Could you check a few things on this model? Use its own coordinates, in mm. Face numbers are marked on the shaded views. A direction names the side the tool comes from. Give positions to 0.01 mm unless a question says otherwise; leave off trailing zeros. Order: outer loops, then holes, each group sorted by start corner. A loop starts at its lowest first (then second) coordinate and runs counter-clockwise, first axis right, second up. Notation, with made-up numbers: (82, -7.75) - (123, -7.75) arc R34 cw to (123, 31.25) - close; hole circle Ø11 at (-27, 17.5). An arc over 180 degrees is marked (long way). One line per question, with ' | ' between items. Start each with the question number.
1. Which directions (+Z, -Z, +X, -X, +Y, -Y) give clear straight access to the entire face, cutting with the end or side of a thin tool? Please do the marked faces 1 and 2.
2. Imagine slicing it at A-A (y = 39.5). Please give me the cut outline in (x, z), and give its area (3 significant figures).
3. Imagine slicing it at B-B (x = 6). Please give me the cut outline in (y, z).
4. For P1, Ø0.8, axis at x = 34, y = 10, coming from the -Z side; P2, Ø8.5, axis at x = 15, y = 15.5, coming from the -Z side; P3, Ø10, axis at y = 46.5, z = -2.5, coming from the -X side; P4, Ø6, axis at x = 6, y = 39.5, coming from the +Z side, each with a flat end and sliding along its axis, tell me the tip position at first contact or that it passes through.
5. I need wall thicknesses on probe 1 along X at (y, z) = (6.5, 3.95); probe 2 along Y at (x, z) = (6, 3.55); probe 3 along X at (y, z) = (45.5, -2.75). Which ranges of each line are inside material? Lowest first, please. Write a range as from..to.
6. Imagine slicing it at C-C (y = 15.5). Please give me the cut outline in (x, z), and give its area (3 significant figures).
7. Imagine slicing it at D-D (z = 3.25). Please give me the cut outline in (x, y), and give its area (3 significant figures).
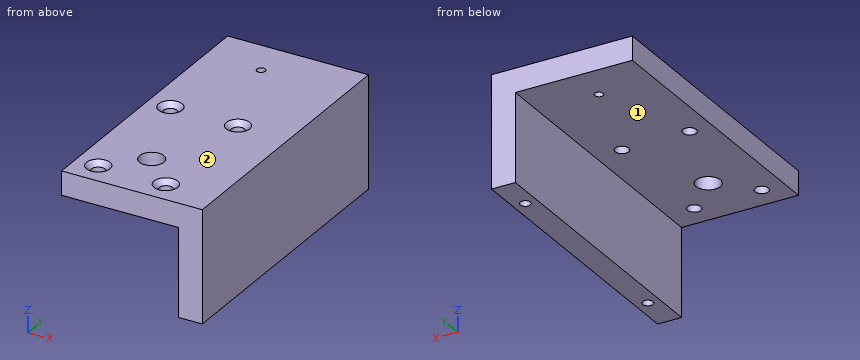
```python
from build123d import *

# Parameters (mm, degrees)
SKETCH1_W                                       = 37.5
SKETCH1_H                                       = 46
SKETCH1_R                                       = 6.25
SKETCH1_R_2                                     = 3.5
SKETCH1_R_3                                     = 3.25
SKETCH1_R_4                                     = 1.7
BOSS_EXTRUDE1_DEPTH                             = 6.35
CSK_FOR_M3_FLAT_HEAD_MACHINE_SCREW1_D           = 3.6
CSK_FOR_M3_FLAT_HEAD_MACHINE_SCREW1_CSINK_D     = 6.3
CSK_FOR_M3_FLAT_HEAD_MACHINE_SCREW1_CSINK_ANGLE = 90
SKETCH3_W                                       = 6.35
SKETCH3_H                                       = 46
BOSS_EXTRUDE2_DEPTH                             = 23.5
BOSS_EXTRUDE4_DEPTH                             = 30
CUT_EXTRUDE1_REACH                              = 91.851
SKETCH6_R                                       = 1.1303
SKETCH7_R                                       = 1.3890625
CUT_EXTRUDE2_DEPTH                              = 10


with BuildPart() as part:
    # Sketch1 → Boss-Extrude1 (new body)
    # profile 1 of 6: a face of its own
    with BuildSketch(Plane.XY):
        with Locations((18.75, 23)):
            Rectangle(SKETCH1_W, SKETCH1_H)
        with Locations((15, 15.5)):
            Circle(SKETCH1_R, mode=Mode.SUBTRACT)
        with Locations((24, 6.5)):
            Circle(SKETCH1_R_2, mode=Mode.SUBTRACT)
        with Locations((6, 6.5)):
            Circle(SKETCH1_R_2, mode=Mode.SUBTRACT)
        with Locations((6, 39.5)):
            Circle(SKETCH1_R_2, mode=Mode.SUBTRACT)
        with Locations((24, 39.5)):
            Circle(SKETCH1_R_2, mode=Mode.SUBTRACT)
    # profile 2 of 6: a face of its own
    with BuildSketch(Plane.XY):
        with Locations((15, 15.5)):
            Circle(SKETCH1_R)
        with Locations((15, 15.5)):
            Circle(SKETCH1_R_3, mode=Mode.SUBTRACT)
    # profile 3 of 6: a face of its own
    with BuildSketch(Plane.XY):
        with Locations((6, 39.5)):
            Circle(SKETCH1_R_2)
        with Locations((6, 39.5)):
            Circle(SKETCH1_R_4, mode=Mode.SUBTRACT)
    # profile 4 of 6: a face of its own
    with BuildSketch(Plane.XY):
        with Locations((24, 39.5)):
            Circle(SKETCH1_R_2)
        with Locations((24, 39.5)):
            Circle(SKETCH1_R_4, mode=Mode.SUBTRACT)
    # profile 5 of 6: a face of its own
    with BuildSketch(Plane.XY):
        with Locations((24, 6.5)):
            Circle(SKETCH1_R_2)
        with Locations((24, 6.5)):
            Circle(SKETCH1_R_4, mode=Mode.SUBTRACT)
    # profile 6 of 6: a face of its own
    with BuildSketch(Plane.XY):
        with Locations((6, 6.5)):
            Circle(SKETCH1_R_2)
        with Locations((6, 6.5)):
            Circle(SKETCH1_R_4, mode=Mode.SUBTRACT)
    extrude(amount=BOSS_EXTRUDE1_DEPTH)

    # CSK for M3 Flat Head Machine Screw1 (through all)
    with Locations(Plane(origin=(6, 6.5, 6.35), x_dir=(1, 0, 0), z_dir=(0, 0, 1))):
        with Locations((0, 0), (0, 33), (18, 33), (18, 0)):
            CounterSinkHole(CSK_FOR_M3_FLAT_HEAD_MACHINE_SCREW1_D / 2, CSK_FOR_M3_FLAT_HEAD_MACHINE_SCREW1_CSINK_D / 2, counter_sink_angle=CSK_FOR_M3_FLAT_HEAD_MACHINE_SCREW1_CSINK_ANGLE)

    # Sketch3 → Boss-Extrude2 (add)
    with BuildSketch(Plane(origin=(0, 0, 0), x_dir=(-1, 0, 0), z_dir=(0, 0, -1))):
        with Locations((-34.325, 23)):
            Rectangle(SKETCH3_W, SKETCH3_H)
    extrude(amount=BOSS_EXTRUDE2_DEPTH)

    # Sketch5 → Boss-Extrude4 (add)
    with BuildSketch(Plane(origin=(0, 46, 0), x_dir=(1, 0, 0), z_dir=(0, 1, 0))):
        Polygon((31.15, 0), (0, 0), (0, -6.35), (37.5, -6.35), (37.5, 23.5), (31.15, 23.5), align=None)
    extrude(amount=BOSS_EXTRUDE4_DEPTH)

    # Sketch6 → Cut-Extrude1 (cut, up to next)
    with BuildSketch(Plane.XY.offset(6.35), mode=Mode.PRIVATE) as cut_extrude1_sk1:
        with Locations((15, 65.5)):
            Circle(SKETCH6_R)
    cut_extrude1_tool1 = extrude(cut_extrude1_sk1.sketch, amount=-CUT_EXTRUDE1_REACH, mode=Mode.PRIVATE) & part.part
    add(cut_extrude1_tool1.solids().sort_by_distance((15, 65.5, 6.35))[0], mode=Mode.SUBTRACT)

    # Sketch7 → Cut-Extrude2 (cut)
    with BuildSketch(Plane(origin=(0, 0, -23.5), x_dir=(-1, 0, 0), z_dir=(0, 0, -1))):
        with Locations((-34.325, 10)):
            Circle(SKETCH7_R)
        with Locations((-34.325, 66)):
            Circle(SKETCH7_R)
    extrude(amount=-CUT_EXTRUDE2_DEPTH, mode=Mode.SUBTRACT)


solid = part.part
```
Results found:
1) face 1: -Z, -X, +Y, -Y | face 2: +Z, +X, -X, +Y, -Y
2) outline: (0, 0) - (4.2, 0) - (4.2, 5) - (2.85, 6.35) - (0, 6.35) - close; (7.8, 0) - (22.2, 0) - (22.2, 5) - (20.85, 6.35) - (9.15, 6.35) - (7.8, 5) - close; (25.8, 0) - (31.15, 0) - (31.15, -23.5) - (37.5, -23.5) - (37.5, 6.35) - (27.15, 6.35) - (25.8, 5) - close | area: 338 mm2
3) outline: (0, 0) - (4.7, 0) - (4.7, 5) - (3.35, 6.35) - (0, 6.35) - close; (8.3, 0) - (37.7, 0) - (37.7, 5) - (36.35, 6.35) - (9.65, 6.35) - (8.3, 5) - close; (41.3, 0) - (76, 0) - (76, 6.35) - (42.65, 6.35) - (41.3, 5) - close
4) P1: stops at z = -13.5 | P2: stops at z = 0 | P3: stops at x = 0 | P4: stops at z = 6.2
5) probe 1: x = 0..4.2, 7.8..22.2, 25.8..37.5 | probe 2: y = 0..4.7, 8.3..37.7, 41.3..76 | probe 3: x = 31.15..37.5
6) outline: (0, 0) - (11.75, 0) - (11.75, 6.35) - (0, 6.35) - close; (18.25, 0) - (31.15, 0) - (31.15, -23.5) - (37.5, -23.5) - (37.5, 6.35) - (18.25, 6.35) - close | area: 346 mm2
7) outline: (0, 0) - (37.5, 0) - (37.5, 76) - (0, 76) - close; hole circle Ø3.6 at (6, 6.5); hole circle Ø3.6 at (6, 39.5); hole circle Ø6.5 at (15, 15.5); hole circle Ø2.26 at (15, 65.5); hole circle Ø3.6 at (24, 6.5); hole circle Ø3.6 at (24, 39.5) | area: 2,770 mm2
